from build123d import *

# Parameters (mm, degrees)
SKETCH1_W           = 30.86
SKETCH1_H           = 42.11
BOSS_EXTRUDE1_DEPTH = 3.25
SKETCH2_OUTSIDE_W   = 43.322
SKETCH2_OUTSIDE_H   = 54.572
SKETCH2_OUTSIDE_W_2 = 25.86
SKETCH2_OUTSIDE_H_2 = 37.11
CUT_EXTRUDE1_DEPTH  = 1.25
FILLET1_R           = 0.25
SKETCH4_W           = 7.1
SKETCH4_H           = 18
CUT_EXTRUDE3_DEPTH  = 27.305140657
SKETCH5_W           = 9.15
SKETCH5_H           = 4
CUT_EXTRUDE4_DEPTH  = 1.25


with BuildPart() as part:
    # Sketch1 → Boss-Extrude1 (new body)
    with BuildSketch(Plane(origin=(0, 0, 0), x_dir=(1, 0, 0), z_dir=(0, 1, 0))):
        Rectangle(SKETCH1_W, SKETCH1_H)
    extrude(amount=BOSS_EXTRUDE1_DEPTH)

    # Sketch2 outside → Cut-Extrude1 (cut)
    with BuildSketch(Plane(origin=(0, 3.25, 0), x_dir=(1, 0, 0), z_dir=(0, 1, 0))):
        Rectangle(SKETCH2_OUTSIDE_W, SKETCH2_OUTSIDE_H)
        Rectangle(SKETCH2_OUTSIDE_W_2, SKETCH2_OUTSIDE_H_2, mode=Mode.SUBTRACT)
    extrude(amount=-CUT_EXTRUDE1_DEPTH, mode=Mode.SUBTRACT)

    # Fillet1
    fillet1_edges = [part.edges().sort_by_distance(p)[0] for p in [
        (15.43, 1, 21.055),
        (-15.43, 1, 21.055),
        (-15.43, 1, -21.055),
        (15.43, 1, -21.055),
        (0, 0, 21.055),
        (-15.43, 0, 0),
        (0, 0, -21.055),
        (15.43, 0, 0),
    ]]
    fillet(fillet1_edges, radius=FILLET1_R)

    # Sketch4 → Cut-Extrude3 (cut, through all)
    with BuildSketch(Plane(origin=(0, 0, 0), x_dir=(-1, 0, 0), z_dir=(0, -1, 0))):
        with Locations((-9.38, 9.555)):
            Rectangle(SKETCH4_W, SKETCH4_H)
    extrude(amount=-CUT_EXTRUDE3_DEPTH, mode=Mode.SUBTRACT)

    # Sketch5 → Cut-Extrude4 (cut)
    with BuildSketch(Plane(origin=(0, 3.25, 0), x_dir=(1, 0, 0), z_dir=(0, 1, 0))):
        with Locations((-8.355, 16.555)):
            Rectangle(SKETCH5_W, SKETCH5_H)
    extrude(amount=-CUT_EXTRUDE4_DEPTH, mode=Mode.SUBTRACT)


solid = part.part
Read the model definition and answer for the solid it produces. Units are mm, in the model's axes. A direction names the side the tool comes from. Round coordinates to 2 decimals unless told otherwise and drop trailing zeros. Write each loop counter-clockwise with the first axis right and the second up, starting at its lowest first coordinate (ties: lowest second). Pieces come first, ordered by that corner, then holes. Notation, with made-up numbers: (25.25, -32.5) - (42.25, -32.5) arc R33 cw to (42.25, 5.5) - close; hole circle Ø5 at (50.25, -27). An arc over 180 degrees is marked (long way). One line per question, with ' | ' between items. Start each with the question number.
1. Section A-A (z = -13.5) is taken. Determine the outline of the cut face in (x, y).
2. Find the intervals of material crossed by probe 1 along Z at (x, y) = (7.5, 0.8) (3 decimals); probe 2 along X at (y, z) = (1.95, -13.5); probe 3 along Y at (x, z) = (13, -13.5), in increasing order. Write a range as [from, to].
3. Section D-D (z = 14) is taken. Determine the outline of the cut face in (x, y), and give its area (3 significant figures).
4. Section C-C (x = 4) is taken. Determine the outline of the cut face in (y, z) (3 decimals), and give its area (3 significant figures).
5. For faces 1 (the face through (12.93, 3, 9)), 2 (the face through (-8, 3, -14.555)), 3 (the face through (9, 2, -0.555)), determine the directions among +Z, -Z, +X, -X, +Y, -Y from which every point of the face is accessible in a straight line to the end or side of a thin tool.
6. Section B-B (y = 1.3) is taken. Determine the outline of the cut face in (x, z) (3 decimals), and give its area (3 significant figures).
7. This flat-tipped pin is pushed along its axis until it touches: pin 1 (0.6 mm diameter, centred on y = 2.5, z = 13.5, fed in from +X). Where does it stop, or does it pass through?
Filled in:
1) outline: (-15.43, 0.25) arc R0.25 ccw to (-15.18, 0) - (5.83, 0) - (5.83, 3.25) - (-12.93, 3.25) - (-12.93, 2) - (-15.43, 2) - close; (12.93, 0) - (15.18, 0) arc R0.25 ccw to (15.43, 0.25) - (15.43, 2) - (12.93, 2) - close
2) probe 1: [-21.055, -18.555], [-0.555, 21.055] | probe 2: [-15.43, 5.83], [12.93, 15.43] | probe 3: [0, 2]
3) outline: (-15.43, 0.25) arc R0.25 ccw to (-15.18, 0) - (15.18, 0) arc R0.25 ccw to (15.43, 0.25) - (15.43, 2) - (12.93, 2) - (12.93, 3.25) - (-12.93, 3.25) - (-12.93, 2) - (-15.43, 2) - close | area: 94.0 mm²
4) outline: (0, -20.805) arc R0.25 ccw to (0.25, -21.055) - (2, -21.055) - (2, -18.555) - (3.25, -18.555) - (3.25, 18.555) - (2, 18.555) - (2, 21.055) - (0.25, 21.055) arc R0.25 ccw to (0, 20.805) - close | area: 131 mm²
5) face 1: +Z, -Z, +X, +Y | face 2: -Z, -X, +Y | face 3: +Y, -Y
6) outline: (-15.43, -20.805) arc R0.25 ccw to (-15.18, -21.055) - (15.18, -21.055) arc R0.25 ccw to (15.43, -20.805) - (15.43, 20.805) arc R0.25 ccw to (15.18, 21.055) - (-15.18, 21.055) arc R0.25 ccw to (-15.43, 20.805) - close; hole (5.83, -18.555) - (12.93, -18.555) - (12.93, -0.555) - (5.83, -0.555) - close | area: 1,170 mm²
7) pin 1: x = 12.93
